```python
from build123d import *

# Parameters (mm, degrees)
SKETCH1_W           = 2.9
SKETCH1_H           = 20
BOSS_EXTRUDE1_DEPTH = 3
CUT_EXTRUDE1_DEPTH  = 4


with BuildPart() as part:
    # Sketch1 → Boss-Extrude1 (new body)
    with BuildSketch(Plane.XY):
        with BuildLine():
            Line((0, 0), (104.9, 0))
            Line((104.9, 0), (104.9, -30))
            Line((104.9, -30), (87.212489335, -40.211889044))
            ThreePointArc((87.212489335, -40.211889044), (52.45, -20), (17.687510665, -40.211889044))
            Line((17.687510665, -40.211889044), (0, -30))
            Line((0, -30), (0, 0))
        make_face()
        with Locations((99.45, -15)):
            Rectangle(SKETCH1_W, SKETCH1_H, mode=Mode.SUBTRACT)
        with Locations((5.45, -15)):
            Rectangle(SKETCH1_W, SKETCH1_H, mode=Mode.SUBTRACT)
    extrude(amount=BOSS_EXTRUDE1_DEPTH)

    # Sketch2 → Cut-Extrude1 (cut, through all)
    with BuildSketch(Plane.XY.offset(3)):
        Polygon((1, 0), (1, -30.577350269), (0, -30), (0, 0), align=None)
        Polygon((103.9, 0), (103.9, -30.577350269), (104.9, -30), (104.9, 0), align=None)
    extrude(amount=-CUT_EXTRUDE1_DEPTH, mode=Mode.SUBTRACT)


solid = part.part
```
Check sheet for the modelled part. Datum: model origin and axes. Units: mm. A direction names the side the tool comes from. Round coordinates to 2 decimals unless told otherwise and drop trailing zeros. Write each loop counter-clockwise with the first axis right and the second up, starting at its lowest first coordinate (ties: lowest second). Pieces come first, ordered by that corner, then holes. Notation, with made-up numbers: (76, -23) -> (84, -23) arc R29 cw to (84, 4) -> close; hole circle Ø9 at (30.5, 34.25). An arc over 180 degrees is marked (long way). One line per question, with ' | ' between items. Start each with the question number.
1. Sectioned sample at B-B, the plane y = -18. Record the cut outline in (x, z).
2. Scan lines: line 1 along X through (y, z) = (-7, 0.95); line 2 along X through (y, z) = (-23.5, 1.35); line 3 along X through (y, z) = (-23, 2.3). Record each from-to range of solid material in increasing order. Write a range as from..to.
3. Sectioned sample at D-D, the plane y = -23.5. Record the cut outline in (x, z).
4. Sectioned sample at C-C, the plane y = -36. Record the cut outline in (x, z), then the cut area to 3 significant figures.
5. Set-up check for faces 1 (the face through (5, -5, 1)), 2 (the face through (53, -15, 0)): record each of +Z, -Z, +X, -X, +Y, -Y from which the full face is reachable in a straight line by a thin tool's end or side.
6. Depth check by flat-ended pin: pin 1 (0.9 mm diameter, centred on x = 99.5, z = 2, fed in from -Y). Enter the tip coordinate at first touch or a pass-through.
7. Release check for a two-part mould opening along X. For faces 3 (the face through (4, -15, 1)), 4 (the face through (9.46, -35.46, 1.48)), 5 (the face through (53, -15, 3)), 6 (the face through (95.67, -35.33, 1.48)) record: +X half, -X half, draft (parallel to the pull), parting line (faces both ways), or undercut.
8. Sectioned sample at A-A, the plane z = 2. Record the cut outline in (x, y), then the cut area to 3 significant figures.
Taken from the geometry:
1) outline: (1, 0) -> (4, 0) -> (4, 3) -> (1, 3) -> close; (6.9, 0) -> (98, 0) -> (98, 3) -> (6.9, 3) -> close; (100.9, 0) -> (103.9, 0) -> (103.9, 3) -> (100.9, 3) -> close
2) line 1: x = 1..4, 6.9..98, 100.9..103.9 | line 2: x = 1..4, 6.9..36.09, 68.81..98, 100.9..103.9 | line 3: x = 1..4, 6.9..37.25, 67.65..98, 100.9..103.9
3) outline: (1, 0) -> (4, 0) -> (4, 3) -> (1, 3) -> close; (6.9, 0) -> (36.09, 0) -> (36.09, 3) -> (6.9, 3) -> close; (68.81, 0) -> (98, 0) -> (98, 3) -> (68.81, 3) -> close; (100.9, 0) -> (103.9, 0) -> (103.9, 3) -> (100.9, 3) -> close
4) outline: (10.39, 0) -> (20.45, 0) -> (20.45, 3) -> (10.39, 3) -> close; (84.45, 0) -> (94.51, 0) -> (94.51, 3) -> (84.45, 3) -> close | area: 60.3 mm^2
5) face 1: +Z, -Z | face 2: -Z, +X, -X, +Y, -Y
6) pin 1: stops at y = -33.38
7) face 3: undercut | face 4: -X half | face 5: draft | face 6: +X half
8) outline: (1, -30.58) -> (17.69, -40.21) arc R40 cw to (87.21, -40.21) -> (103.9, -30.58) -> (103.9, 0) -> (1, 0) -> close; hole (4, -25) -> (6.9, -25) -> (6.9, -5) -> (4, -5) -> close; hole (98, -25) -> (100.9, -25) -> (100.9, -5) -> (98, -5) -> close | area: 2,860 mm^2
